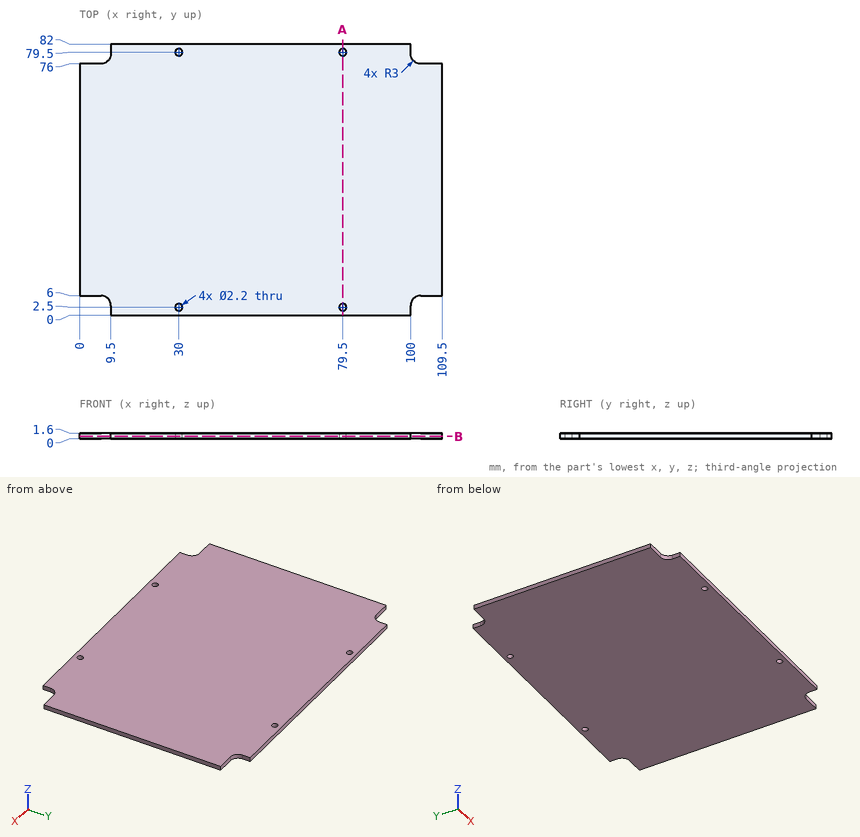
Study the drawing (mm; zero at the part's minimum x, y, z) and answer. Give positions to 0.01 mm unless a question says otherwise; leave off trailing zeros. Order: outer loops, then holes, each group sorted by start corner. A loop starts at its lowest first (then second) coordinate and runs counter-clockwise, first axis right, second up.
1. Section A-A, the plane x = 79.5 is taken. Determine the outline of the cut face in (y, z).
Result sheet:
outline: (0, 0) - (1.4, 0) - (1.4, 1.6) - (0, 1.6) - close; (3.6, 0) - (78.4, 0) - (78.4, 1.6) - (3.6, 1.6) - close; (80.6, 0) - (82, 0) - (82, 1.6) - (80.6, 1.6) - close
2. Straight lines are drawn through the part: L1, parallel to Y at x = 30, z = 0.6; L2, parallel to X at y = 79.5, z = 1.2; L3, parallel to Y at x = 6.5, z = 1.05. For each, find the intervals that lie inside material, in ascending order.
Result sheet:
L1: y = 0 to 1.4, 3.6 to 78.4, 80.6 to 82
L2: x = 9.5 to 28.9, 31.1 to 78.4, 80.6 to 100
L3: y = 6 to 76
3. Section B-B, the plane z = 0.75 is taken. Determine the outline of the cut face in (x, y), and give its area (3 significant figures).
Result sheet:
outline: (0, 6) - (6.5, 6) arc R3 cw to (9.5, 3) - (9.5, 0) - (100, 0) - (100, 3) arc R3 cw to (103, 6) - (109.5, 6) - (109.5, 76) - (103, 76) arc R3 cw to (100, 79) - (100, 82) - (9.5, 82) - (9.5, 79) arc R3 cw to (6.5, 76) - (0, 76) - close; hole circle Ø2.2 at (30, 2.5); hole circle Ø2.2 at (30, 79.5); hole circle Ø2.2 at (79.5, 2.5); hole circle Ø2.2 at (79.5, 79.5)
area: 8,740 mm2
4. Each of these flat-tipped pins is pushed along its axis until it touches: P1, Ø2, axis at x = 79.5, y = 2.5, coming from the -Z side; P2, Ø0.5, axis at y = 80, z = 1, coming from the -X side; P3, Ø8, axis at x = 24.5, y = 27, coming from the -Z side; P4, Ø0.5, axis at x = 2, z = 1, coming from the -Y side. Where does it stop, or does it pass through?
Result sheet:
P1: passes through
P2: stops at x = 9.5
P3: stops at z = 0
P4: stops at y = 6
